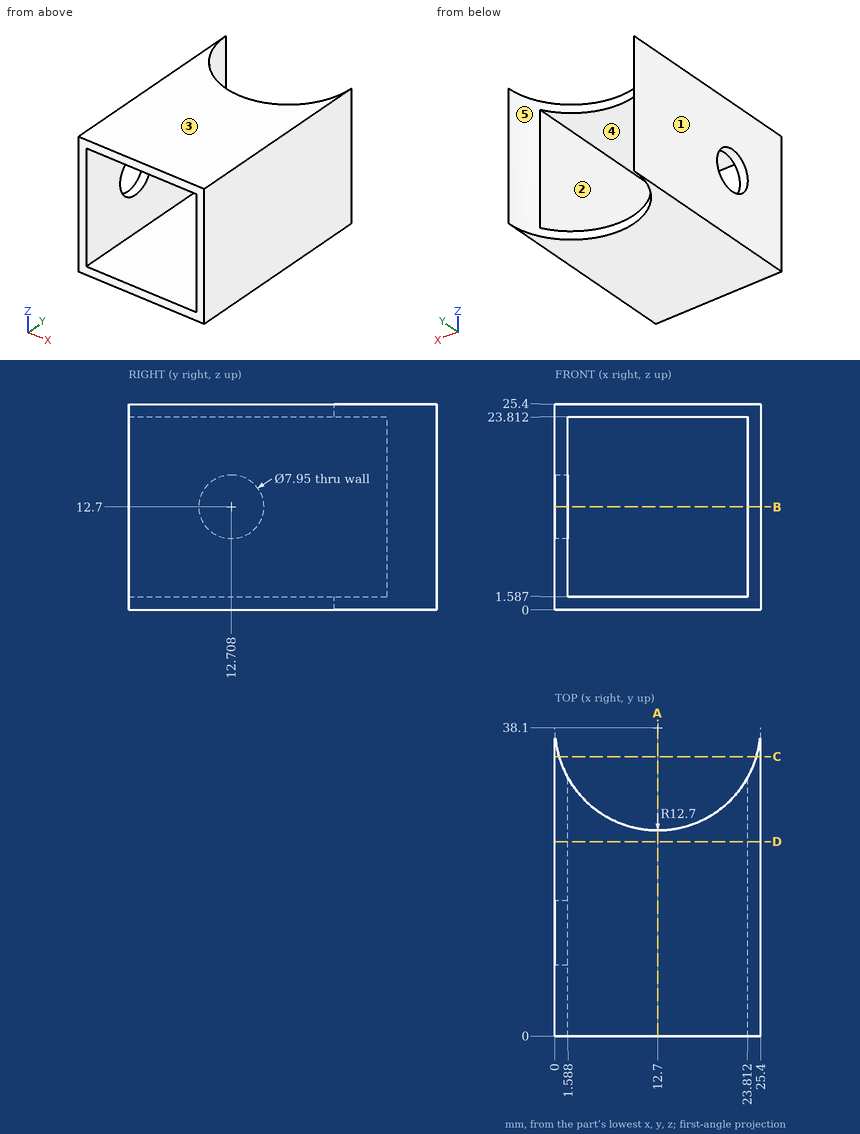
Part print with two shaded views. Sizes in mm from the minimum x, y, z corner. A direction names the side the tool comes from. Round coordinates to 2 decimals unless told otherwise and drop trailing zeros. Loops run counter-clockwise (first coordinate to the right, second up) from the corner with the lowest first, then second, coordinate; pieces in that order, holes last. Notation, with made-up numbers: (21, 10) - (51, 10) arc R26 cw to (51, 27) - close; hole circle Ø9 at (-8, 33). An arc over 180 degrees is marked (long way). Put each result on its own line as item: value.
1. Wall check: line 1 (X direction, y = 31, z = 15.25); line 2 (Y direction, x = 1, z = 12.7) (1 decimal). Give the ranges that are in metal, low to high.
Geometry check:
line 1: 0 to 1.59, 23.81 to 25.4
line 2: 0 to 8.7, 16.7 to 33.2
2. 3-axis set-ups, long thin cutter, end or side, ignore diameter. For the marked faces 4 and 5: which of +Z, -Z, +X, -X, +Y, -Y reach the whole face in a straight line?
Geometry check:
face 4: +Y, -Y
face 5: +Z, -Z, +Y
3. Two-plate mould, pull along Z, no slides. Class the marked faces 1, 2 and 3: released by +Z, released by -Z, zero draft, split by the parting line, or undercut.
Geometry check:
face 1: zero draft
face 2: undercut
face 3: released by +Z
4. Slice it at D-D on y = 24. List the corners of the cut face in (x, z).
Geometry check:
outline: (0, 0) - (25.4, 0) - (25.4, 25.4) - (0, 25.4) - close; hole (1.59, 1.59) - (23.81, 1.59) - (23.81, 23.81) - (1.59, 23.81) - close
5. Pin check, flat tip, straight feed: P1, Ø2, axis at x = 21.5, y = 31.5, coming from the -Z side. Stop position of the tip, or through.
Geometry check:
P1: through
6. Slice it at B-B on z = 12.7. List the corners of the cut face in (x, y).
Geometry check:
outline: (0, 0) - (1.59, 0) - (1.59, 8.73) - (0, 8.73) - close; (0, 16.68) - (1.59, 16.68) - (1.59, 31.95) arc R12.7 cw to (0, 38.1) - close; (23.81, 0) - (25.4, 0) - (25.4, 38.1) arc R12.7 cw to (23.81, 31.95) - close
7. Slice it at C-C on y = 34.5. List the corners of the cut face in (x, z).
Geometry check:
outline: (0, 0) - (0.52, 0) - (0.52, 25.4) - (0, 25.4) - close; (24.88, 0) - (25.4, 0) - (25.4, 25.4) - (24.88, 25.4) - close
8. Slice it at A-A on x = 12.7. List the corners of the cut face in (y, z).
Geometry check:
outline: (0, 0) - (25.4, 0) - (25.4, 1.59) - (0, 1.59) - close; (0, 23.81) - (25.4, 23.81) - (25.4, 25.4) - (0, 25.4) - close
